```python
from build123d import *

# Parameters (mm, degrees)
F0_W      = 46.2659336627
F0_H      = 37.4186895788
F1_DEPTH  = 16
F2_DEPTH  = 396
F3_DEPTH  = 396
F4_W      = 286.636531353
F4_H      = 292.4217879772
F5_DEPTH  = 5
F7_DEPTH  = 5
F8_DEPTH  = 24.58
F9_DEPTH  = 28.59
F10_DEPTH = 44.51
F11_DEPTH = 43.6
F12_DEPTH = 23.54
F13_DEPTH = 25.39
F14_DEPTH = 8.54
F15_DEPTH = 6.68
F16_DEPTH = 6.68
F17_DEPTH = 6.68
F18_DEPTH = 1.72
F19_DEPTH = 11
F20_R     = 3


with BuildPart() as f1:
    # F0 (on Front) → F1 (new body)
    with BuildSketch(Plane.XZ):
        with Locations((23.1329668313, 18.7093447894)):
            Rectangle(F0_W, F0_H)
    extrude(amount=F1_DEPTH)

    # F2 (add): a face of the model
    f2_faces = [f1.faces().sort_by_distance(p)[0] for p in [
        (0, -8, 18.7093447894),
    ]]
    extrude(f2_faces, amount=-F2_DEPTH)

    # F3 (add): a face of the model
    f3_faces = [f1.faces().sort_by_distance(p)[0] for p in [
        (198, -8, 0),
    ]]
    extrude(f3_faces, amount=-F3_DEPTH)

    # F4 (on face) → F5 (cut)
    with BuildSketch(Plane.XZ.offset(16)):
        with Locations((194.2568123341, 201.971784234)):
            Rectangle(F4_W, F4_H)
    extrude(amount=-F5_DEPTH, mode=Mode.SUBTRACT)

    # F6 (on face) → F7 (join)
    with BuildSketch(Plane.XZ.offset(11)):
        Polygon((211.1129611731, 348.1826782227), (162.3977422714, 348.1826782227), (162.3977422714, 257.6956450939), (50.9385466576, 257.6956450939), (50.9385466576, 215.037047863), (160.5494618416, 215.037047863), (160.5494618416, 55.7608902454), (207.5308859348, 55.7608902454), (207.5308859348, 219.3460762501), (337.5750780106, 219.3460762501), (337.5750780106, 256.7791342735), (211.1129611731, 256.7791342735), align=None)
    extrude(amount=F7_DEPTH)

    # F8 (add): a face of the model
    f8_faces = [f1.faces().sort_by_distance(p)[0] for p in [
        (105.7440042496, -13.5, 215.037047863),
    ]]
    extrude(f8_faces, amount=F8_DEPTH)

    # F9 (add): a face of the model
    f9_faces = [f1.faces().sort_by_distance(p)[0] for p in [
        (272.5529819727, -13.5, 219.3460762501),
    ]]
    extrude(f9_faces, amount=F9_DEPTH)

    # F10 (cut): a face of the model
    f10_faces = [f1.faces().sort_by_distance(p)[0] for p in [
        (106.6681444645, -13.5, 257.6956450939),
    ]]
    extrude(f10_faces, amount=-F10_DEPTH, mode=Mode.SUBTRACT)

    # F11 (cut): a face of the model
    f11_faces = [f1.faces().sort_by_distance(p)[0] for p in [
        (274.3440195918, -13.5, 256.7791342735),
    ]]
    extrude(f11_faces, amount=-F11_DEPTH, mode=Mode.SUBTRACT)

    # F12 (cut): a face of the model
    f12_faces = [f1.faces().sort_by_distance(p)[0] for p in [
        (162.3977422714, -13.5, 280.6841616583),
    ]]
    extrude(f12_faces, amount=-F12_DEPTH, mode=Mode.SUBTRACT)

    # F13 (cut): a face of the model
    f13_faces = [f1.faces().sort_by_distance(p)[0] for p in [
        (160.5494618416, -13.5, 123.1089690542),
    ]]
    extrude(f13_faces, amount=-F13_DEPTH, mode=Mode.SUBTRACT)

    # F14 (cut): a face of the model
    f14_faces = [f1.faces().sort_by_distance(p)[0] for p in [
        (211.1129611731, -13.5, 280.6809062481),
    ]]
    extrude(f14_faces, amount=-F14_DEPTH, mode=Mode.SUBTRACT)

    # F15 (add): a face of the model
    f15_faces = [f1.faces().sort_by_distance(p)[0] for p in [
        (185.9377422714, -13.5, 280.6841616583),
    ]]
    extrude(f15_faces, amount=F15_DEPTH)

    # F16 (add): a face of the model
    f16_faces = [f1.faces().sort_by_distance(p)[0] for p in [
        (202.5729611731, -13.5, 280.6809062481),
    ]]
    extrude(f16_faces, amount=F16_DEPTH)

    # F17 (add): a face of the model
    f17_faces = [f1.faces().sort_by_distance(p)[0] for p in [
        (185.9394618416, -13.5, 123.1089690542),
    ]]
    extrude(f17_faces, amount=F17_DEPTH)

    # F18 (add): a face of the model
    f18_faces = [f1.faces().sort_by_distance(p)[0] for p in [
        (207.5308859348, -13.5, 123.2584832478),
    ]]
    extrude(f18_faces, amount=F18_DEPTH)

    # F19 (cut): faces of the model
    f19_faces = [f1.faces().sort_by_distance(p)[0] for p in [
        (115.0990042496, -11, 123.1089690542),
        (273.4140195918, -11, 280.6809062481),
        (273.4129819727, -11, 123.2584832478),
        (115.0981444645, -11, 280.6841616583),
    ]]
    extrude(f19_faces, amount=-F19_DEPTH, mode=Mode.SUBTRACT)

    # F20
    f20_edges = [f1.edges().sort_by_distance(p)[0] for p in [
        (0, -16, 198),
        (198, -16, 0),
        (396, -16, 198),
        (198, -16, 396),
        (50.938547, -16, 123.108969),
        (115.099004, -16, 190.457048),
        (179.259462, -16, 123.108969),
        (115.099004, -16, 55.76089),
        (273.412982, -16, 55.76089),
        (209.250886, -16, 123.258483),
        (273.412982, -16, 190.756076),
        (337.575078, -16, 123.258483),
        (115.098144, -16, 348.182678),
        (179.257742, -16, 280.684162),
        (115.098144, -16, 213.185645),
        (50.938547, -16, 280.684162),
        (273.41402, -16, 348.182678),
        (337.575078, -16, 280.680906),
        (273.41402, -16, 213.179134),
        (209.252961, -16, 280.680906),
    ]]
    fillet(f20_edges, radius=F20_R)


solid = f1.part
```
Design review of the part built by this model. Coordinates are the model's own, in mm. A direction names the side the tool comes from. Coordinates: 2 decimals unless noted, no trailing zeros. Loops run counter-clockwise (first coordinate to the right, second up) from the corner with the lowest first, then second, coordinate; pieces in that order, holes last. Notation, with made-up numbers: (43.5, -19.75) - (64.5, -19.75) arc R21 cw to (64.5, -10.75) - close; hole circle Ø6 at (21.5, 56). An arc over 180 degrees is marked (long way). Use CSV: the item, a comma, the result in double quotes. Start each with the question number.
1) Wall thickness on L1, parallel to X at y = -9.75, z = 61.5; L2, parallel to Z at x = 153, y = -11.75; L3, parallel to Z at x = 310.5, y = -1.5: over which ranges is each line inside the solid? List them lowest first. Write a range as from..to.
2) Consider section C-C on y = -6.25. Write out the cut boundary in (x, z), then the cut area to 3 significant figures.
3) The part is to be moulded in two halves that separate along Z. For faces 1 (the flat face through (337.575, -7, 122)), 2 (the flat face through (114, -7, 55.761)), 3 (the flat face through (195, -16, 195)), 4 (the flat face through (195, -6, 396)), say which applies: +Z half, -Z half, draft (parallel to the pull), parting line (faces both ways), or undercut.
4) Consider section A-A on x = 103.5. Write out the cut boundary in (y, z), then the cut area to 3 significant figures.
5) Consider section B-B on z = 260. Write out the cut boundary in (x, y), then the cut area to 3 significant figures.
6) Tool access review of faces 5 (the flat face through (195, 0, 201)), 6 (the flat face through (50.939, -6, 282)): name each direction out of +Z, -Z, +X, -X, +Y, -Y from which nothing blocks a thin tool from reaching the whole face with its end or side.
Geometry says:
1,L1,"0..50.94, 179.26..209.25, 337.58..396"
1,L2,"0..55.76, 190.46..213.19, 348.18..396"
1,L3,"0..55.76, 190.76..213.18, 348.18..396"
2,outline,"(0, 0) - (396, 0) - (396, 396) - (0, 396) - close; hole (50.94, 55.76) - (179.26, 55.76) - (179.26, 190.46) - (50.94, 190.46) - close; hole (50.94, 213.19) - (179.26, 213.19) - (179.26, 348.18) - (50.94, 348.18) - close; hole (209.25, 55.76) - (337.58, 55.76) - (337.58, 190.76) - (209.25, 190.76) - close; hole (209.25, 213.18) - (337.58, 213.18) - (337.58, 348.18) - (209.25, 348.18) - close"
2,area,"87,600 mm^2"
3,face 1,"undercut"
3,face 2,"undercut"
3,face 3,"draft"
3,face 4,"+Z half"
4,outline,"(-16, 3) arc R3 ccw to (-13, 0) - (0, 0) - (0, 55.76) - (-13, 55.76) arc R3 ccw to (-16, 52.76) - close; (-16, 193.46) arc R3 ccw to (-13, 190.46) - (0, 190.46) - (0, 213.19) - (-13, 213.19) arc R3 ccw to (-16, 210.19) - close; (-16, 351.18) arc R3 ccw to (-13, 348.18) - (0, 348.18) - (0, 396) - (-13, 396) arc R3 ccw to (-16, 393) - close"
4,area,"2,010 mm^2"
5,outline,"(0, -13) arc R3 ccw to (3, -16) - (47.94, -16) arc R3 ccw to (50.94, -13) - (50.94, 0) - (0, 0) - close; (179.26, -13) arc R3 ccw to (182.26, -16) - (206.25, -16) arc R3 ccw to (209.25, -13) - (209.25, 0) - (179.26, 0) - close; (337.58, -13) arc R3 ccw to (340.58, -16) - (393, -16) arc R3 ccw to (396, -13) - (396, 0) - (337.58, 0) - close"
5,area,"2,220 mm^2"
6,face 5,"+Z, -Z, +X, -X, +Y"
6,face 6,"+Y, -Y"
